Check sheet for the drawn part. Datum: minimum x, y, z corner. Units: mm. Coordinates: 2 decimals unless noted, no trailing zeros. Write each loop counter-clockwise with the first axis right and the second up, starting at its lowest first coordinate (ties: lowest second). Pieces come first, ordered by that corner, then holes. Notation, with made-up numbers: M 11,71 L 45,71 A23 ccw 45,109 Z; hole C 44.5,37.5 d10. An arc over 180 degrees is marked long. Answer in a Markdown table with one row per item.
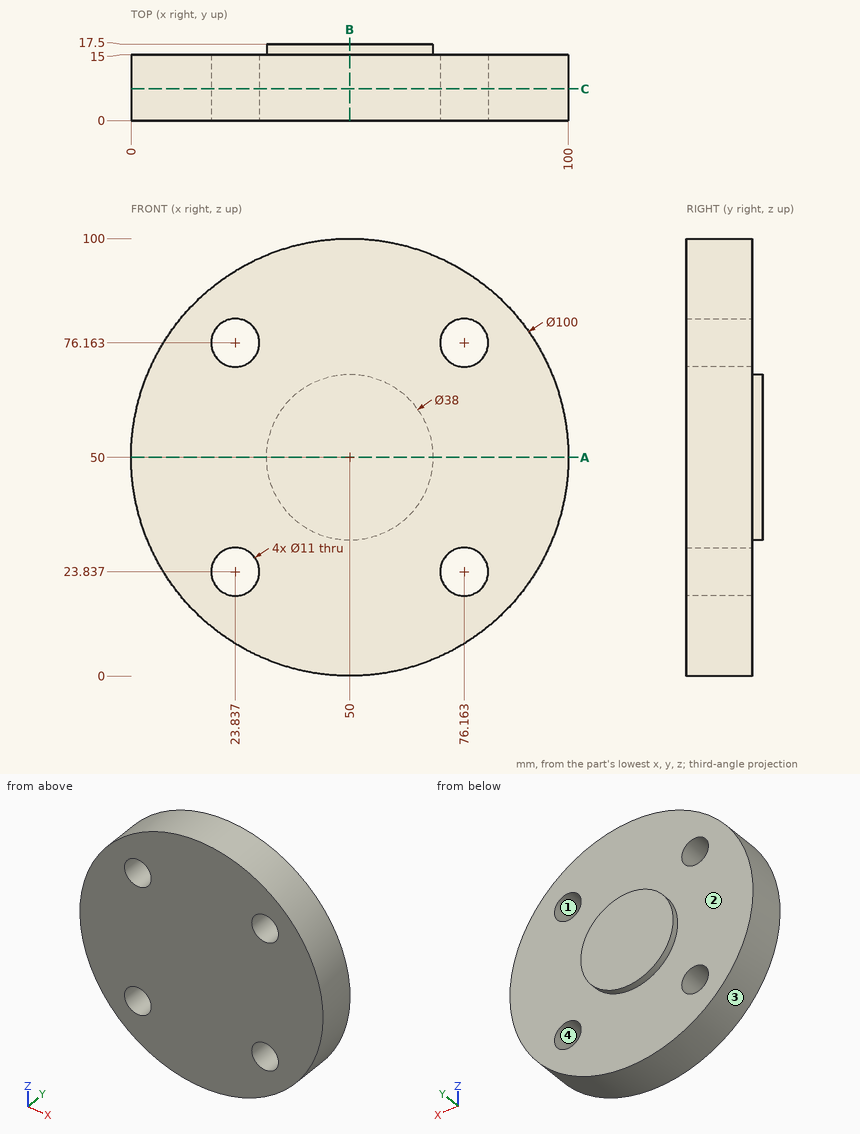
1) Release check for a two-part mould opening along X. For the marked faces 1, 2, 3 and 4 record: +X half, -X half, draft (parallel to the pull), parting line (faces both ways), or undercut.
Response values:
| item | result |
|---|---|
| face 1 | undercut |
| face 2 | draft |
| face 3 | parting line |
| face 4 | undercut |
2) Thickness scan on L1, parallel to Z at x = 22, y = 6; L2, parallel to X at y = 7.5, z = 80.5 (1 decimal); L3, parallel to X at y = 7.75, z = 74. Record the ranges inside material, lowest first. Write a range as [from, to].
Response values:
| item | result |
|---|---|
| L1 | z = [8.58, 18.65], [29.02, 70.98], [81.35, 91.42] |
| L2 | x = [10.4, 20.5], [27.2, 72.8], [79.5, 89.6] |
| L3 | x = [6.14, 18.78], [28.89, 71.11], [81.22, 93.86] |
3) Depth check by flat-ended pin: pin 1 (12.5 mm diameter, centred on x = 76.16, z = 23.84, fed in from +Y); pin 2 (14.5 mm diameter, centred on x = 76.16, z = 76.16, fed in from -Y); pin 3 (5 mm diameter, centred on y = 9.5, z = 27.5, fed in from -X); pin 4 (10 mm diameter, centred on x = 58, y = 3.5, fed in from +Z). Enter the tip coordinate at first touch or a pass-through.
Response values:
| item | result |
|---|---|
| pin 1 | stops at y = 15 |
| pin 2 | stops at y = 0 |
| pin 3 | stops at x = 4.17 |
| pin 4 | stops at z = 99.91 |
4) Sectioned sample at C-C (y = 7.25). Record the cut outline in (x, z).
Response values:
| item | result |
|---|---|
| outline | C 50,50 d100; hole C 23.84,23.84 d11; hole C 23.84,76.16 d11; hole C 76.16,23.84 d11; hole C 76.16,76.16 d11 |
5) Sectioned sample at A-A (z = 50). Record the cut outline in (x, y).
Response values:
| item | result |
|---|---|
| outline | M 0,0 L 100,0 L 100,15 L 69,15 L 69,17.5 L 31,17.5 L 31,15 L 0,15 Z |
6) Sectioned sample at B-B (x = 50). Record the cut outline in (y, z).
Response values:
| item | result |
|---|---|
| outline | M 0,0 L 15,0 L 15,31 L 17.5,31 L 17.5,69 L 15,69 L 15,100 L 0,100 Z |
